Build history of the part. All positions in model axes, mm. A direction names the side the tool comes from. Give positions to 0.01 mm unless a question says otherwise; leave off trailing zeros. Write each loop counter-clockwise with the first axis right and the second up, starting at its lowest first coordinate (ties: lowest second). Pieces come first, ordered by that corner, then holes. Notation, with made-up numbers: (-23, 29.5) -> (21, 29.5) arc R8 ccw to (21, 36.5) -> close; hole circle Ø4 at (63, -18.5). An arc over 180 degrees is marked (long way). Put each result on its own line as item: value.
from build123d import *

# Parameters (mm, degrees)
BOSS_EXTRUDE1_DEPTH     = 50.8
SKETCH6_R               = 2.4892
CUT_EXTRUDE2_DEPTH      = 23.225
CUT_EXTRUDE2_DEPTH_BACK = 4.175
SKETCH5_R               = 2.4892
CUT_EXTRUDE1_DEPTH      = 24.8125


with BuildPart() as part:
    # Sketch1 → Boss-Extrude1 (new body)
    with BuildSketch(Plane(origin=(0, 0, 0), x_dir=(1, 0, 0), z_dir=(0, 1, 0))):
        Polygon((0, 0), (25.4, 0), (25.4, 23.8125), (22.225, 23.8125), (22.225, 3.175), (3.175, 3.175), (3.175, 23.8125), (0, 23.8125), align=None)
    extrude(amount=BOSS_EXTRUDE1_DEPTH)

    # Sketch6 → Cut-Extrude2 (cut, two sides)
    with BuildSketch(Plane(origin=(3.175, 0, 0), x_dir=(0, 0, -1), z_dir=(1, 0, 0))) as cut_extrude2_sk:
        with Locations((13.49375, 12.7)):
            Circle(SKETCH6_R)
        with Locations((13.49375, 38.1)):
            Circle(SKETCH6_R)
    extrude(amount=CUT_EXTRUDE2_DEPTH, mode=Mode.SUBTRACT)
    extrude(cut_extrude2_sk.sketch, amount=-CUT_EXTRUDE2_DEPTH_BACK, mode=Mode.SUBTRACT)

    # Sketch5 → Cut-Extrude1 (cut, through all)
    with BuildSketch(Plane.XY):
        with Locations((12.7, 44.45)):
            Circle(SKETCH5_R)
        with Locations((12.7, 31.75)):
            Circle(SKETCH5_R)
    extrude(amount=-CUT_EXTRUDE1_DEPTH, mode=Mode.SUBTRACT)


solid = part.part
1) Slice it at B-B (y = 38.1). Write the cut outline in (x, z) (1 decimal).
Filled sheet:
outline: (0, -23.8) -> (3.2, -23.8) -> (3.2, -16) -> (0, -16) -> close; (0, -11) -> (3.2, -11) -> (3.2, -3.2) -> (22.2, -3.2) -> (22.2, -11) -> (25.4, -11) -> (25.4, 0) -> (0, 0) -> close; (22.2, -23.8) -> (25.4, -23.8) -> (25.4, -16) -> (22.2, -16) -> close
2) Pin check, flat tip, straight feed: pin 1 (9.5 mm diameter, centred on x = 12, y = 34.5, fed in from -Z) (3 decimals). Stop position of the tip, or through.
Filled sheet:
pin 1: z = -3.175
3) Slice it at D-D (y = 44.45). Write the cut outline in (x, z) (1 decimal).
Filled sheet:
outline: (0, -23.8) -> (3.2, -23.8) -> (3.2, -3.2) -> (10.2, -3.2) -> (10.2, 0) -> (0, 0) -> close; (15.2, -3.2) -> (22.2, -3.2) -> (22.2, -23.8) -> (25.4, -23.8) -> (25.4, 0) -> (15.2, 0) -> close
4) Pull direction Z, two halves, no side cores. Call faces 1 (the flat face through (15, 0, -3)), 2 (the flat face through (24, 25, -23.812)), 3 (the cylindrical face through (23.79, 35.67, -12.95)): released by +Z, released by -Z, zero draft, split by the parting line, or undercut.
Filled sheet:
face 1: zero draft
face 2: released by -Z
face 3: undercut
5) Wall check: L1, parallel to X at y = 25, z = -4 (3 decimals); L2, parallel to Y at x = 12.7, z = -0.65; L3, parallel to Z at x = 6.5, y = 13.5 (3 decimals). Give the ranges that are in metal, low to high.
Filled sheet:
L1: 0 to 3.175, 22.225 to 25.4
L2: 0 to 29.26, 34.24 to 41.96, 46.94 to 50.8
L3: -3.175 to 0
6) Tool access for faces 4 (the flat face through (22.225, 25, -14)), 5 (the cylindrical face through (10.213, 31.859, -1.565)): list every direction of +Z, -Z, +X, -X, +Y, -Y with a clear straight run to the whole face (end or side of a thin tool).
Filled sheet:
face 4: -Z, +Y, -Y
face 5: +Z, -Z
7) Slice it at A-A (z = -17.25). Write the cut outline in (x, y) (3 decimals), plus the area to 3 significant figures.
Filled sheet:
outline: (0, 0) -> (3.175, 0) -> (3.175, 50.8) -> (0, 50.8) -> close; (22.225, 0) -> (25.4, 0) -> (25.4, 50.8) -> (22.225, 50.8) -> close
area: 323 mm2
8) Slice it at C-C (x = 12.7). Write the cut outline in (y, z) (3 decimals).
Filled sheet:
outline: (0, -3.175) -> (29.261, -3.175) -> (29.261, 0) -> (0, 0) -> close; (34.239, -3.175) -> (41.961, -3.175) -> (41.961, 0) -> (34.239, 0) -> close; (46.939, -3.175) -> (50.8, -3.175) -> (50.8, 0) -> (46.939, 0) -> close
